from build123d import *

# Parameters (mm, degrees)
F0_W     = 29
F0_H     = 16.5
F1_DEPTH = 38.5
F2_T     = -2
F3_DEPTH = 2.25
F4_SIZE  = 1.99999
F6_DEPTH = 25


# Not quite as in the source:
# - a fillet or chamfer is up to 0.001 mm smaller than in the source, because OpenCascade refuses the exact size


with BuildPart() as f1:
    # F0 (on Top) → F1 (new body)
    with BuildSketch(Plane.XY):
        with Locations((14.5, 8.25)):
            Rectangle(F0_W, F0_H)
    extrude(amount=F1_DEPTH)

    # F2
    f2_openings = [f1.faces().sort_by_distance(p)[0] for p in [
        (14.5, 8.25, 38.5),
    ]]
    offset(amount=F2_T, openings=f2_openings)

    # F3 (add): a face of the model
    f3_faces = [f1.faces().sort_by_distance(p)[0] for p in [
        (14.5, 8.25, 0),
    ]]
    extrude(f3_faces, amount=F3_DEPTH)

    # F4 (size 2 in the source; OpenCascade refuses exactly that, so slightly less here)
    f4_edges = [f1.edges().sort_by_distance(p)[0] for p in [
        (29, 0, 18.125),
        (0, 0, 18.125),
        (14.5, 0, 38.5),
        (14.5, 0, -2.25),
    ]]
    chamfer(f4_edges, length=F4_SIZE)

    # F5 (on face) → F6 (cut)
    with BuildSketch(Plane.XZ):
        Polygon((17.364, 10.584), (12.635, 10.584), (6.464, 6.414), (6.464, 2.69), (23.536, 2.69), (23.536, 6.414), align=None)
    extrude(amount=-F6_DEPTH, mode=Mode.SUBTRACT)


solid = f1.part
For this review, take the finished solid that the model builds, in its own axes (mm). A direction names the side the tool comes from. Give positions to 0.01 mm unless a question says otherwise; leave off trailing zeros. Loops run counter-clockwise (first coordinate to the right, second up) from the corner with the lowest first, then second, coordinate; pieces in that order, holes last. Notation, with made-up numbers: M 8,80.25 L 57,80.25 A28 ccw 57,102.25 Z; hole C 47.25,34.5 d11. An arc over 180 degrees is marked long. Answer as a JSON object with one key per item and string values. Group by question number.
Q1. Mouldability with a two-part tool opening along X and no side actions: class faces 1 (the flat face through (14, 16.5, 18)), 2 (the flat face through (28, 1, 18)), 3 (the flat face through (23.536, 15, 5)) as +X half, -X half, draft (parallel to the pull), parting line (faces both ways), or undercut.
Q2. Insertion check: P1, Ø1, axis at x = 18.5, y = 3.5, coming from the +Z side; P2, Ø2, axis at x = 14, y = 0.5, coming from the -Z side; P3, Ø0.6, axis at x = 17.5, y = 1.5, coming from the +Z side. Each pin has a flat end and moves straight along its axis. Give the tip position at first contact, or say it passes through.
Q3. Add section B-B on x = 18.75. Give the number of separate pieces and of enclosed holes in the cut face, and give its area (3 significant figures).
Q4. Add section C-C on z = 29. Give the boundary of the cut face in (x, y).
Q5. For probe 1 along X at (y, z) = (7, 5.5); probe 2 along Y at (x, z) = (3, 32.5); probe 3 along Z at (x, y) = (5, 7.5), list the stretches that pass through material, from the lowest coordinate up. Write a range as [from, to].
Q6. Add section A-A on y = 15. Give the boundary of the cut face in (x, z) (3 decimals), and give its area (3 significant figures).
Q7. Tool access review of faces 4 (the flat face through (14, 15, 38.5)), 5 (the flat face through (15, 1, 2.69)), 6 (the flat face through (14, 2, 24)): name each direction out of +Z, -Z, +X, -X, +Y, -Y from which nothing blocks a thin tool from reaching the whole face with its end or side.
Checked values:
{
 "1": {"face 1": "draft", "face 2": "+X half", "face 3": "undercut"},
 "2": {"P1": "z = 2", "P2": "z = -1.75", "P3": "z = 38.3"},
 "3": {"separate pieces": "3", "enclosed holes": "0", "area": "184 mm²"},
 "4": {"outline": "M 0,2 L 2,0 L 27,0 L 29,2 L 29,16.5 L 0,16.5 Z; hole M 2,2 L 27,2 L 27,14.5 L 2,14.5 Z"},
 "5": {"probe 1": "[0, 2], [27, 29]", "probe 2": "[0, 2], [14.5, 16.5]", "probe 3": "[-2.25, 2]"},
 "6": {"outline": "M 0,-2.25 L 29,-2.25 L 29,38.5 L 0,38.5 Z; hole M 6.464,2.69 L 23.536,2.69 L 23.536,6.414 L 17.364,10.584 L 12.635,10.584 L 6.464,6.414 Z", "area": "1,070 mm²"},
 "7": {"face 4": "+Z, +X, -X, +Y, -Y", "face 5": "+Y, -Y", "face 6": "+Z"}
}
